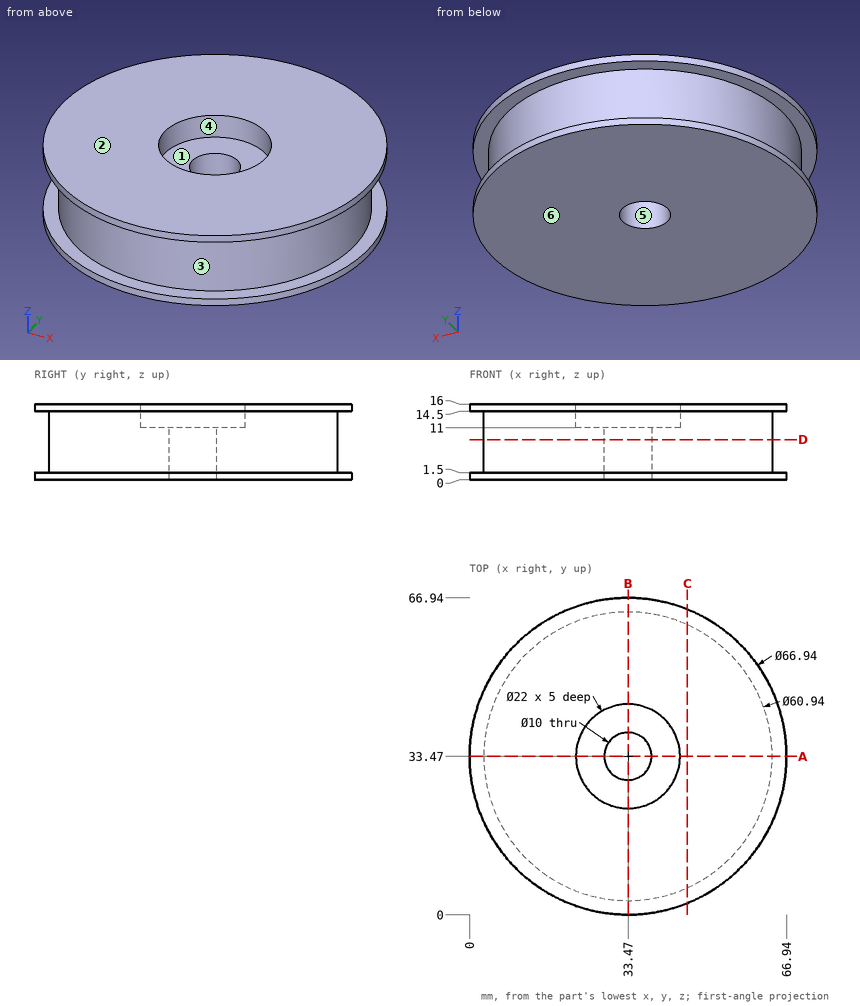
Drawing for the job (mm, zero at the part's lowest x, y, z). A direction names the side the tool comes from. Coordinates: 2 decimals unless noted, no trailing zeros. Write each loop counter-clockwise with the first axis right and the second up, starting at its lowest first coordinate (ties: lowest second). Pieces come first, ordered by that corner, then holes. Notation, with made-up numbers: (14, 2) - (41, 2) arc R35 ccw to (41, 35) - close; hole circle Ø8 at (-12, -1.75). An arc over 180 degrees is marked (long way). Write each question's results on one line, items separated by ' | '. Start each with the question number.
1) Probe line 1 along Y through (x, z) = (33.47, 8.25); line 2 along Y through (x, z) = (33.47, 12); line 3 along Z through (x, y) = (6, 17). List the from-to ranges inside material, lowest first. Write a range as from..to.
2) Flat gauge pins, fed straight in: P1, Ø1.5, axis at x = 37.5, z = 7.5, coming from the +Y side; P2, Ø1, axis at y = 22, z = 11, coming from the +X side; P3, Ø6, axis at x = 12.5, z = 10.5, coming from the +Y side. Where does each tip first touch, or does it go through?
3) 3-axis set-ups, long thin cutter, end or side, ignore diameter. For the marked faces 1 and 2: which of +Z, -Z, +X, -X, +Y, -Y reach the whole face in a straight line?
4) Cut at C-C (x = 46). Write the cut outline in (y, z), then the cut area to 3 significant figures.
5) Mould opens along Y. For the marked faces 3, 4, 5 and 6 say: pulls with the +Y half, pulls with the -Y half, needs draft (parallel to the pull), parting line crosses it, or undercut.
6) Cut at D-D (z = 8.5). Write the cut outline in (x, y), then the cut area to 3 significant figures.
7) Cut at A-A (y = 33.47). Write the cut outline in (x, z), then the cut area to 3 significant figures.
Returned:
1) line 1: 3..28.47, 38.47..63.94 | line 2: 3..22.47, 44.47..63.94 | line 3: 0..1.5, 14.5..16
2) P1: y = 63.76 | P2: x = 61.9 | P3: y = 58.08
3) face 1: +Z | face 2: +Z, +X, -X, +Y, -Y
4) outline: (2.43, 0) - (64.51, 0) - (64.51, 1.5) - (61.24, 1.5) - (61.24, 14.5) - (64.51, 14.5) - (64.51, 16) - (2.43, 16) - (2.43, 14.5) - (5.7, 14.5) - (5.7, 1.5) - (2.43, 1.5) - close | area: 908 mm^2
5) face 3: parting line crosses it | face 4: undercut | face 5: undercut | face 6: needs draft
6) outline: circle Ø60.94 at (33.47, 33.47); hole circle Ø10 at (33.47, 33.47) | area: 2,840 mm^2
7) outline: (0, 0) - (28.47, 0) - (28.47, 11) - (22.47, 11) - (22.47, 16) - (0, 16) - (0, 14.5) - (3, 14.5) - (3, 1.5) - (0, 1.5) - close; (38.47, 0) - (66.94, 0) - (66.94, 1.5) - (63.94, 1.5) - (63.94, 14.5) - (66.94, 14.5) - (66.94, 16) - (44.47, 16) - (44.47, 11) - (38.47, 11) - close | area: 773 mm^2
